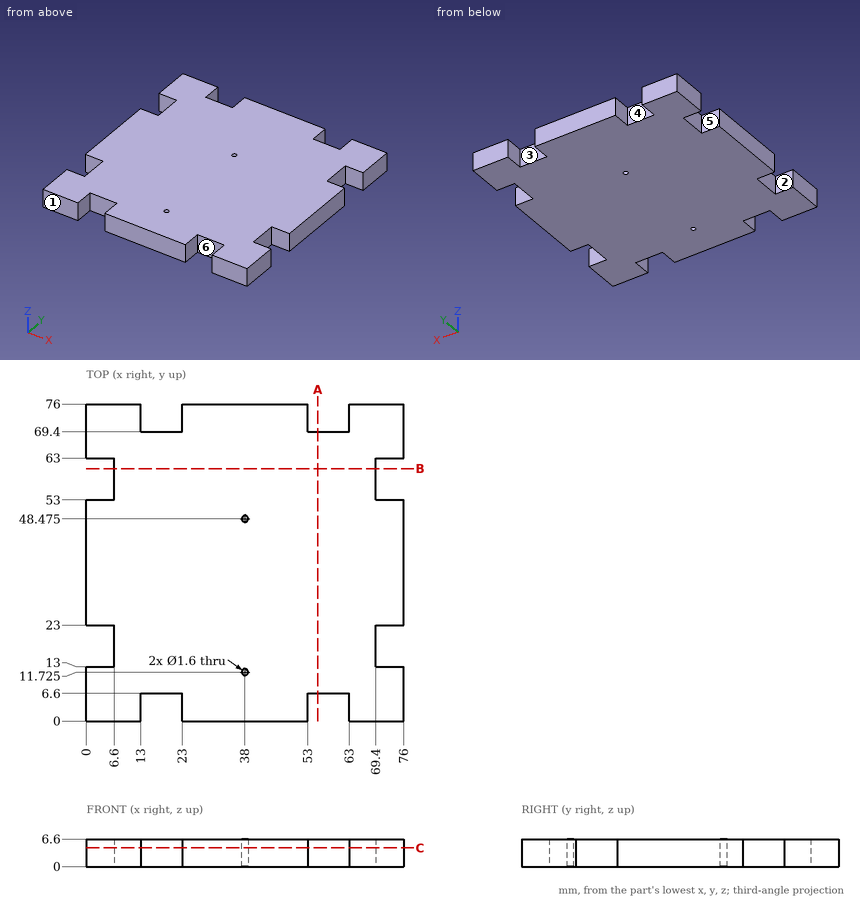
Part print with two shaded views. Sizes in mm from the minimum x, y, z corner. A direction names the side the tool comes from. Round coordinates to 2 decimals unless told otherwise and drop trailing zeros. Write each loop counter-clockwise with the first axis right and the second up, starting at its lowest first coordinate (ties: lowest second). Pieces come first, ordered by that corner, then holes. Notation, with made-up numbers: (-17, 86) -> (-5, 86) arc R25 ccw to (-5, 110) -> close; hole circle Ø9 at (-10.5, 88). An arc over 180 degrees is marked (long way). Put each result on its own line as item: value.
Item 1: Slice it at A-A, the plane x = 55.5. Give the cut face in (y, z).
Here are the results:
outline: (6.6, 0) -> (69.4, 0) -> (69.4, 6.6) -> (6.6, 6.6) -> close
Item 2: Flat gauge pins, fed straight in: P1, Ø3.5, axis at y = 18, z = 3.5, coming from the +X side; P2, Ø2, axis at x = 16, z = 2.5, coming from the -Y side; P3, Ø2, axis at y = 19.5, z = 2.5, coming from the -X side. Where does each tip first touch, or does it go through?
Here are the results:
P1: stops at x = 69.4
P2: stops at y = 6.6
P3: stops at x = 6.6
Item 3: Two-plate mould, pull along Y, no slides. Class the marked faces 1, 2 and 3: pulls with the +Y half, pulls with the -Y half, needs draft (parallel to the pull), parting line crosses it, or undercut.
Here are the results:
face 1: pulls with the -Y half
face 2: undercut
face 3: pulls with the +Y half
Item 4: Slice it at C-C, the plane z = 4.5. Count the separate pieces of the cut face and the enclosed holes in it, plus the area to 3 significant figures.
Here are the results:
separate pieces: 1
enclosed holes: 2
area: 5,240 mm^2
Item 5: Tool access for the marked faces 4, 5 and 6: list every direction of +Z, -Z, +X, -X, +Y, -Y with a clear straight run to the whole face (end or side of a thin tool).
Here are the results:
face 4: +Z, -Z, +Y
face 5: +Z, -Z, -X
face 6: +Z, -Z, -Y
Item 6: Wall check: probe 1 along Y at (x, z) = (38, 2.25) (3 decimals); probe 2 along Y at (x, z) = (3.5, 1). Give the ranges that are in metal, low to high. Write a range as from..to.
Here are the results:
probe 1: y = 0..10.925, 12.525..47.675, 49.275..76
probe 2: y = 0..13, 23..53, 63..76
